Autodesk Inventor part; units mm, degrees
ref_plane "Work Plane1" through (4, 0, 0) normal (0, 0.5, 0.866) x (1, 0, 0)
ref_plane "YZ Plane" through (0, 0, 0) normal (1, 0, 0) x (0, 1, 0)
ref_plane "XZ Plane" through (0, 0, 0) normal (0, 1, 0) x (-1, 0, 0)
sketch "Sketch1" plane through (0, 0, 0) normal (0, 0, 1) x (1, 0, 0)
  line L0 (0, 0) -> (5.5, 0)
  line L1 (8, 0.866) -> (8, 1.5)
  line L2 (8, 1.5) -> (0, 1.5)
  line L3 (8, 0.866) -> (6, 0.866)
  line L4 (6, 0.866) -> (5.5, 0)
  line L5 (0, -0.3) -> (0, 1.8)
  line L6 (0, 1.5) -> (0, 0)
  dimension "d0" = 2
  dimension "d1" = 60
  dimension "d2" = 3
  dimension "d3" = 1.7321
  dimension "d5" = 8
revolve "Body" add sketch "Sketch1" angle 360 about axis through (0, 0, 0) along (1, 0, 0)
chamfer "Chamfer1" distance 0.3067 angle 45 1 edges at (8, -1.5, 0) measured on face at (8, 1.2658, -0.1887)
sketch "Sketch2" plane through (8, 0, 0) normal (1, 0, 0) x (0, 0, -1)
  circle A0 centre (0, 0) radius 0.866
  line L0 (-0.433, 0.75) -> (0.433, 0.75)
  line L1 (0.433, 0.75) -> (0.866, 0)
  line L2 (0.866, 0) -> (0.433, -0.75)
  line L3 (0.433, -0.75) -> (-0.433, -0.75)
  line L4 (-0.433, -0.75) -> (-0.866, 0)
  line L5 (-0.866, 0) -> (-0.433, 0.75)
extrude "Slot" add sketch "Sketch2" against normal up to next contours L1 A0 | A0 L2 | L0 A0 | A0 L3 | L5 A0 | A0 L4
thread "Thread"
chamfer "Chamfer2" distance 0.3067 angle 45 1 edges at (0, -1.5, 0) measured on face at (2.5644, 1.4806, -0.2406)
ref_plane "Work Plane1" through (4, 0, 0) normal (0, 0.5, 0.866) x (1, 0, 0)
equation "\"d0\" = INTI"
equation "\"d2\" = NND"
equation "\"d3\" = 1.1547 * SW"
equation "\"d5\" = NLG"
equation "\"d7\" = -0.5 * GD1 + 0.5 * NND"
equation "\"d8\" = FAWI"
equation "\"d29\" = -0.5 * GD1 + 0.5 * NND"
equation "\"d11\" = NLG"
equation "\"d13\" = -0.5 * GD1 + 0.5 * NND"
equation "\"d14\" = FAWI"
equation "\"d30\" = -0.5 * GD1 + 0.5 * NND"
equation "\"NND\" = 3"
equation "\"NLG\" = 8"
equation "\"INTI\" = 2"
equation "\"FAWI\" = 45deg"
equation "\"SW\" = 1.5"
equation "\"GD1\" = THREADDIA - 1.2269 * PTC"
equation "\"FAWI1\" = 45deg"
equation "\"GUL\" = 0.61345 * PTC"
equation "\"SPD\" = 2"
equation "\"SEWI\" = 90deg"
equation "\"TOA\" = 30deg"
equation "\"THREADDIA\" = 3"
equation "\"PTC\" = 0.5"
equation "\"GAL\" = 0.61345 * PTC"
equation "\"E0\" = 1.155 * SW"
properties part number "ISO 4026 - M3 x 8" material "Stainless Steel, 440C"
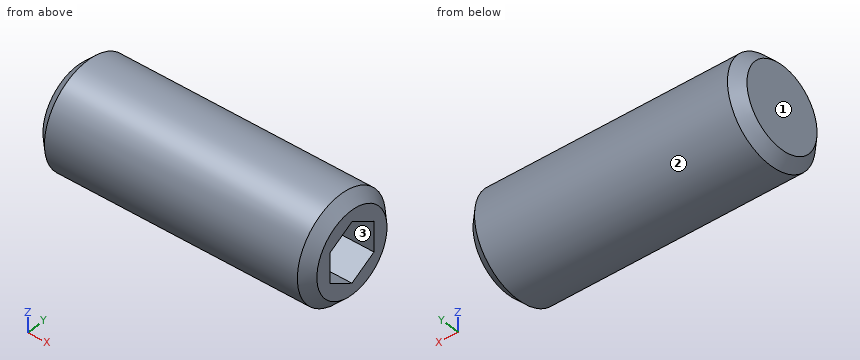
Design review of the part built by this model. Coordinates are the model's own, in mm. Face numbers are marked on the shaded views. Coordinates: 2 decimals unless noted, no trailing zeros. Order: outer loops, then holes, each group sorted by start corner. A loop starts at its lowest first (then second) coordinate and runs counter-clockwise, first axis right, second up. Notation, with made-up numbers: M 21,79 L 58,79 A21 cw 58,90 Z; hole C 61.25,9.25 d2. An arc over 180 degrees is marked long. Use a Markdown table: item, result.
(1) Add section B-B (x = 2.75). Give the boundary of the cut face in (y, z), then the cut area to 3 significant figures.
Worked answers:
| item | result |
|---|---|
| outline | C 0,0 d3 |
| area | 7.07 mm2 |
(2) For P1, Ø1, axis at x = 1, y = -1, coming from the -Z side; P2, Ø1.5, axis at x = 6, y = 1, coming from the -Z side, all flat-tipped, find the tip position at first contact; note any pin that passes through.
Worked answers:
| item | result |
|---|---|
| P1 | stops at z = -1.41 |
| P2 | stops at z = -1.48 |
(3) Draft analysis for pull direction Y (two halves, no side actions). For the marked faces 1, 2 and 3, state which applies: released by +Y, released by -Y, zero draft, split by the parting line, or undercut.
Worked answers:
| item | result |
|---|---|
| face 1 | zero draft |
| face 2 | split by the parting line |
| face 3 | undercut |
(4) Wall thickness on probe 1 along Y at (x, z) = (1, -1.3); probe 2 along Y at (x, z) = (6.5, -0.2); probe 3 along Z at (x, y) = (7, -0.3): over which ranges is each line inside the solid? List them lowest first.
Worked answers:
| item | result |
|---|---|
| probe 1 | y = -0.75 to 0.75 |
| probe 2 | y = -1.49 to -0.75, 0.75 to 1.49 |
| probe 3 | z = -1.47 to -0.69, 0.69 to 1.47 |
(5) Add section A-A (x = 7.25). Give the boundary of the cut face in (y, z), then the cut area to 3 significant figures.
Worked answers:
| item | result |
|---|---|
| outline | C 0,0 d3; hole M -0.75,-0.43 L 0,-0.87 L 0.75,-0.43 L 0.75,0.43 L 0,0.87 L -0.75,0.43 Z |
| area | 5.12 mm2 |
